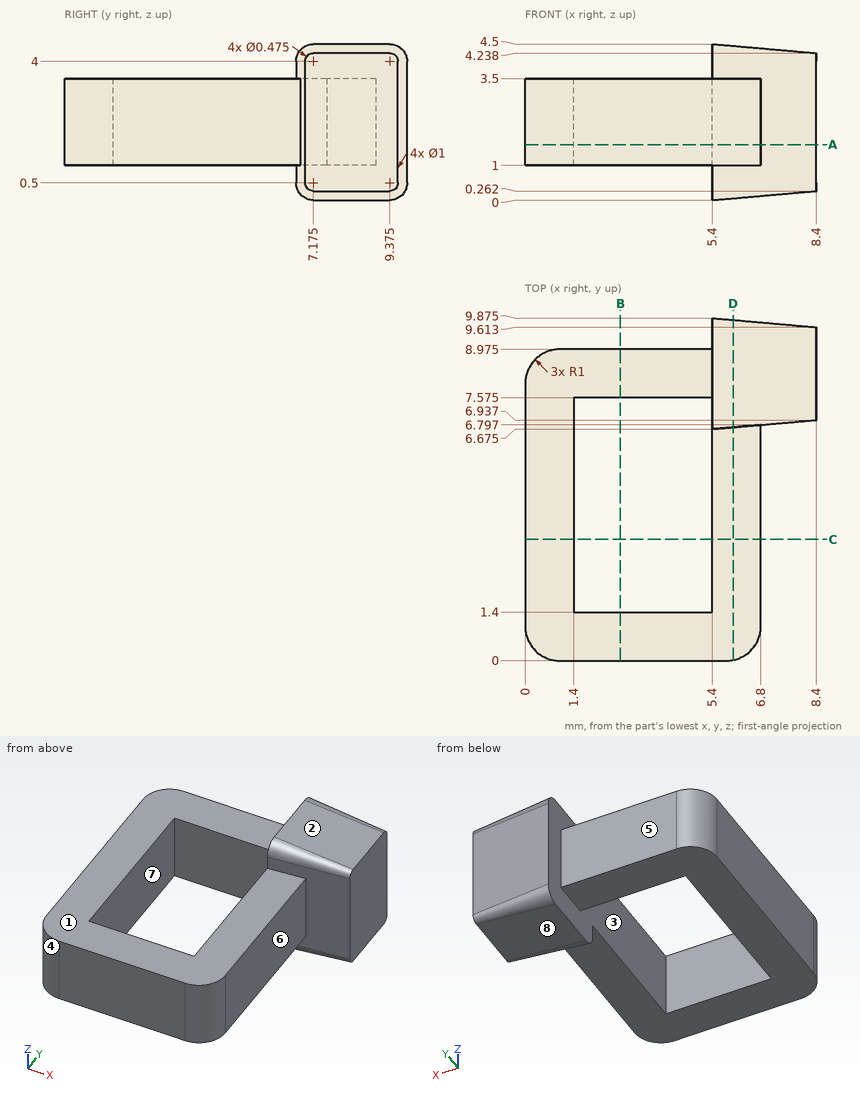
Can you work these out from the drawing? Everything is in mm from the part's minimum corner. A direction names the side the tool comes from. Give positions to 0.01 mm unless a question says otherwise; leave off trailing zeros. Loops run counter-clockwise (first coordinate to the right, second up) from the corner with the lowest first, then second, coordinate; pieces in that order, holes last. Notation, with made-up numbers: (20.25, -6.75) -> (30.25, -6.75) arc R27 ccw to (30.25, 11.25) -> close; hole circle Ø2 at (-28, -34.75). An arc over 180 degrees is marked (long way). Return JSON: item names as keys, results as strings.
Q1. For pin 1 Ø2 at (x, y) = (4.5, 3.5) entering from +Z; pin 2 Ø1.5 at (x, z) = (7, 1) entering from -Y; pin 3 Ø2 at (x, z) = (4, 1.5) entering from +Y (1 decimal), each with a flat end and sliding along its axis, tell me the tip position at first contact or that it passes through.
Checks:
{"pin 1": "stops at z = 3.5", "pin 2": "stops at y = 0.11", "pin 3": "stops at y = 9"}
Q2. I need wall thicknesses on probe 1 along X at (y, z) = (5.5, 1.7); probe 2 along Y at (x, z) = (4.75, 3.45) (1 decimal); probe 3 along X at (y, z) = (7.25, 0.3). Which ranges of each line are inside material? Lowest first, please.
Checks:
{"probe 1": "x = 0 to 1.4, 5.4 to 6.8", "probe 2": "y = 0 to 1.4, 7.6 to 9", "probe 3": "x = 5.4 to 8.4"}
Q3. We'd pull the mould along X, two halves only. Please class the marked faces 1, 2, 3 and 4: released by +X, released by -X, zero draft, split by the parting line, or undercut.
Checks:
{"face 1": "zero draft", "face 2": "released by +X", "face 3": "undercut", "face 4": "released by -X"}
Q4. On a 3-axis mill with a long thin cutter (end or side, diameter ignored), from which of +Z, -Z, +X, -X, +Y, -Y can I reach the whole of each face in a straight line? I mean the marked faces 5, 6, 7 and 8. Say none if no direction works.
Checks:
{"face 5": "+Z, -Z, -X, +Y", "face 6": "+Z, -Z, +X, -Y", "face 7": "+Z, -Z", "face 8": "-Z, +X, +Y, -Y"}
Q5. I want a section at B-B, the plane x = 2.75. List the corners of the cut face in (y, z) for me (1 decimal).
Checks:
{"outline": "(0, 1) -> (1.4, 1) -> (1.4, 3.5) -> (0, 3.5) -> close; (7.6, 1) -> (9, 1) -> (9, 3.5) -> (7.6, 3.5) -> close"}
Q6. I want a section at A-A, the plane z = 1.6. List the corners of the cut face in (x, y) for me (1 decimal).
Checks:
{"outline": "(0, 1) arc R1 ccw to (1, 0) -> (5.8, 0) arc R1 ccw to (6.8, 1) -> (6.8, 6.8) -> (8.4, 6.9) -> (8.4, 9.6) -> (5.4, 9.9) -> (5.4, 9) -> (1, 9) arc R1 ccw to (0, 8) -> close; hole (1.4, 1.4) -> (5.4, 1.4) -> (5.4, 7.6) -> (1.4, 7.6) -> close"}
Q7. I want a section at C-C, the plane y = 3.5. List the corners of the cut face in (x, z) for me.
Checks:
{"outline": "(0, 1) -> (1.4, 1) -> (1.4, 3.5) -> (0, 3.5) -> close; (5.4, 1) -> (6.8, 1) -> (6.8, 3.5) -> (5.4, 3.5) -> close"}
Q8. I want a section at D-D, the plane x = 6. List the corners of the cut face in (y, z) for me (1 decimal), then the cut area to 3 significant figures.
Checks:
{"outline": "(0, 1) -> (6.7, 1) -> (6.7, 0.5) arc R0.4 ccw to (7.2, 0.1) -> (9.4, 0.1) arc R0.4 ccw to (9.8, 0.5) -> (9.8, 4) arc R0.4 ccw to (9.4, 4.4) -> (7.2, 4.4) arc R0.4 ccw to (6.7, 4) -> (6.7, 3.5) -> (0, 3.5) -> close", "area": "30.2 mm2"}
